from build123d import *

# Parameters (mm, degrees)
F1_DEPTH = 2


with BuildPart() as f1:
    # F0 (on Top) → F1 (new body)
    with BuildSketch(Plane.XY):
        Polygon((2, 6.481428), (0, 6.481428), (-2, 6.481428), (-4, -6.518572), (0, -6.518572), (4, -6.518572), align=None)
        Polygon((-2.599652, -2.499616), (-2.133971, -2.499616), (-2.064983, -5.771744), (-3.14582, -5.777694), align=None, mode=Mode.SUBTRACT)
        Polygon((-1.338938, -5.800603), (-1.338938, -2.499616), (-0.466865, -2.499616), (-0.483132, -5.800603), align=None, mode=Mode.SUBTRACT)
        Polygon((-2.522781, -1.629516), (-2.104775, 0.564183), (-2.0927, -1.629516), align=None, mode=Mode.SUBTRACT)
        Polygon((-1.354969, -1.629516), (-1.338938, 1.325562), (-0.483132, 1.325562), (-0.466865, -1.629516), align=None, mode=Mode.SUBTRACT)
        Polygon((1.338938, -5.800603), (0.483132, -5.800603), (0.466865, -2.499616), (1.338938, -2.499616), align=None, mode=Mode.SUBTRACT)
        Polygon((2.599652, -2.499616), (3.14582, -5.777694), (2.064983, -5.771744), (2.133971, -2.499616), align=None, mode=Mode.SUBTRACT)
        Polygon((1.354969, -1.629516), (0.466865, -1.629516), (0.483132, 1.325562), (1.338938, 1.325562), align=None, mode=Mode.SUBTRACT)
        Polygon((2.522781, -1.629516), (2.0927, -1.629516), (2.104775, 0.564183), align=None, mode=Mode.SUBTRACT)
        Polygon((-1.34072, 5.643583), (-0.483132, 5.643583), (-0.464214, 2.206922), (-1.34072, 2.206922), align=None, mode=Mode.SUBTRACT)
        Polygon((1.34072, 5.643583), (1.34072, 2.206922), (0.464214, 2.206922), (0.483132, 5.643583), align=None, mode=Mode.SUBTRACT)
    extrude(amount=F1_DEPTH)


solid = f1.part
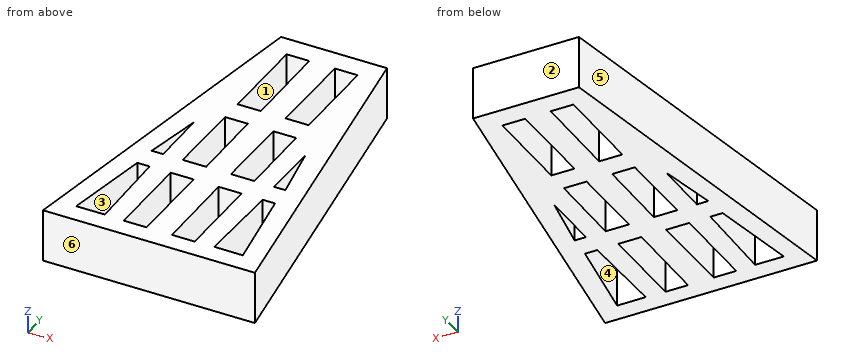
The model under review builds one solid part; all positions refer to its coordinate system, in mm. Face numbers are marked on the shaded views. A direction names the side the tool comes from. Give positions to 0.01 mm unless a question says otherwise; leave off trailing zeros. Write each loop counter-clockwise with the first axis right and the second up, starting at its lowest first coordinate (ties: lowest second). Pieces come first, ordered by that corner, then holes. Notation, with made-up numbers: M 9.5,71.5 L 36.5,71.5 A22 ccw 36.5,88.5 Z; hole C 56,23.25 d2. An arc over 180 degrees is marked long. One line per question, with ' | ' between items. Start each with the question number.
Item 1: Draft analysis for pull direction Y (two halves, no side actions). For the marked faces 3, 4, 5 and 6, state which applies: released by +Y, released by -Y, zero draft, split by the parting line, or undercut.
Item 2: For the marked faces 1 and 2, list the 3-axis set-ups (+Z, -Z, +X, -X, +Y, -Y) from which the entire face can be reached by the end or side of a thin tool; tool diameter is ignored.
Item 3: We need section C-C on x = 3. Write out the cut boundary in (y, z), plus the area to 3 significant figures.
Item 4: We need section D-D on y = -1. Write out the cut boundary in (x, z), plus the area to 3 significant figures.
Item 5: For pin 1 (1 mm diameter, centred on y = -3.5, z = 1.5, fed in from +X); pin 2 (0.6 mm diameter, centred on y = -4.5, z = 0.5, fed in from -X), all flat-tipped, find the tip position at first contact; note any pin that passes through.
Item 6: Wall thickness on line 1 (X direction, y = -4.5, z = 1.85); line 2 (X direction, y = 4, z = 1.15); line 3 (X direction, y = -0.25, z = 0.45): over which ranges is each line inside the solid? List them lowest first. Write a range as from..to.
Item 7: We need section B-B on y = 4. Write out the cut boundary in (x, z).
Item 8: We need section A-A on x = -1. Write out the cut boundary in (y, z), plus the area to 3 significant figures.
Results found:
1) face 3: undercut | face 4: undercut | face 5: released by +Y | face 6: released by -Y
2) face 1: +Z, -Z | face 2: +Z, -Z, +X, -X, +Y
3) outline: M -6.52,0 L -5.78,0 L -5.78,2 L -6.52,2 Z; M -4.9,0 L -0.02,0 L -0.02,2 L -4.9,2 Z | area: 11.3 mm2
4) outline: M -3.15,0 L -2.4,0 L -2.4,2 L -3.15,2 Z; M -2.1,0 L -1.35,0 L -1.35,2 L -2.1,2 Z; M -0.47,0 L 0.47,0 L 0.47,2 L -0.47,2 Z; M 1.35,0 L 2.1,0 L 2.1,2 L 1.35,2 Z; M 2.4,0 L 3.15,0 L 3.15,2 L 2.4,2 Z | area: 7.85 mm2
5) pin 1: stops at x = 3.61 | pin 2: stops at x = -3.74
6) line 1: x = -3.69..-2.93, -2.09..-1.34, -0.48..0.48, 1.34..2.09, 2.93..3.69 | line 2: x = -2.38..-1.34, -0.47..0.47, 1.34..2.38 | line 3: x = -3.04..-2.26, -2.1..-1.35, -0.47..0.47, 1.35..2.1, 2.26..3.04
7) outline: M -2.38,0 L -1.34,0 L -1.34,2 L -2.38,2 Z; M -0.47,0 L 0.47,0 L 0.47,2 L -0.47,2 Z; M 1.34,0 L 2.38,0 L 2.38,2 L 1.34,2 Z
8) outline: M -6.52,0 L -5.8,0 L -5.8,2 L -6.52,2 Z; M -2.5,0 L -1.63,0 L -1.63,2 L -2.5,2 Z; M 1.33,0 L 2.21,0 L 2.21,2 L 1.33,2 Z; M 5.64,0 L 6.48,0 L 6.48,2 L 5.64,2 Z | area: 6.61 mm2
